Work out the finished part from the listing and answer in its coordinate system (mm). Face numbers are marked on the shaded views. Coordinates: 2 decimals unless noted, no trailing zeros. Write each loop counter-clockwise with the first axis right and the second up, starting at its lowest first coordinate (ties: lowest second). Pieces come first, ordered by that corner, then holes. Notation, with made-up numbers: (46, -24) - (66, -24) arc R21 ccw to (66, 12) - close; hole circle Ø6 at (0, 39). An arc over 180 degrees is marked (long way). One line per item, written item: value.
```python
from build123d import *

# Parameters (mm, degrees)
ESQUISSE1_W             = 92.6
ESQUISSE1_H             = 142.6
BASE_EXTRUSION_DEPTH    = 7
ESQUISSE4_R             = 1.6
ENL_V_MAT_EXTRU_2_DEPTH = 108.918117107
ESQUISSE2_W             = 79.5
ESQUISSE2_H             = 104
ENL_V_MAT_EXTRU_3_DEPTH = 4
ESQUISSE6_W             = 86.3
ESQUISSE6_H             = 9.5
ENL_V_MAT_EXTRU_4_DEPTH = 4
ESQUISSE7_W             = 120
ESQUISSE7_H             = 17.9
ENL_V_MAT_EXTRU_6_DEPTH = 4
ESQUISSE8_W             = 13.8
ESQUISSE8_H             = 8.9
ESQUISSE8_W_2           = 65.8
ENL_V_MAT_EXTRU_7_DEPTH = 15


with BuildPart() as part:
    # Esquisse1 → Base-Extrusion (new body)
    with BuildSketch(Plane.XY):
        with Locations((1.3, -25.3)):
            Rectangle(ESQUISSE1_W, ESQUISSE1_H)
    extrude(amount=BASE_EXTRUSION_DEPTH)

    # Esquisse4 → Enlèv. mat.-Extru.2 (cut, through all)
    with BuildSketch(Plane.XY.offset(7)):
        with Locations((-30.2, 44)):
            Circle(ESQUISSE4_R)
        with Locations((43.6, 44)):
            Circle(ESQUISSE4_R)
        with Locations((-30.2, -94.6)):
            Circle(ESQUISSE4_R)
        with Locations((43.6, -94.6)):
            Circle(ESQUISSE4_R)
    extrude(amount=-ENL_V_MAT_EXTRU_2_DEPTH, mode=Mode.SUBTRACT)

    # Esquisse2 → Enlèv. mat.-Extru.3 (cut)
    with BuildSketch(Plane.XY.offset(7)):
        with Locations((5.05, -15.3)):
            Rectangle(ESQUISSE2_W, ESQUISSE2_H)
    extrude(amount=-ENL_V_MAT_EXTRU_3_DEPTH, mode=Mode.SUBTRACT)

    # Esquisse6 → Enlèv. mat.-Extru.4 (cut)
    with BuildSketch(Plane.XY.offset(7)):
        with Locations((7.85, 44.25)):
            Rectangle(ESQUISSE6_W, ESQUISSE6_H)
    extrude(amount=-ENL_V_MAT_EXTRU_4_DEPTH, mode=Mode.SUBTRACT)

    # Esquisse7 → Enlèv. mat.-Extru.6 (cut)
    with BuildSketch(Plane.XY.offset(7)):
        with Locations((0, -99.05)):
            Rectangle(ESQUISSE7_W, ESQUISSE7_H)
    extrude(amount=-ENL_V_MAT_EXTRU_6_DEPTH, mode=Mode.SUBTRACT)

    # Esquisse8 → Enlèv. mat.-Extru.7 (cut)
    with BuildSketch(Plane(origin=(0, 0, 0), x_dir=(-1, 0, 0), z_dir=(0, 0, -1))):
        with Locations((41.1, -94.55)):
            Rectangle(ESQUISSE8_W, ESQUISSE8_H)
        with Locations((-6.7, -94.55)):
            Rectangle(ESQUISSE8_W_2, ESQUISSE8_H)
    extrude(amount=-ENL_V_MAT_EXTRU_7_DEPTH, mode=Mode.SUBTRACT)


solid = part.part
```
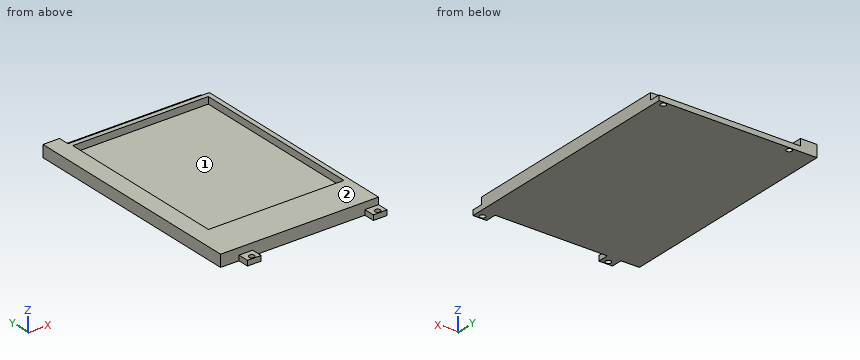
Item 1: Section D-D, the plane z = 1.75 is taken. Determine the outline of the cut face in (x, y), then the cut area to 3 significant figures.
Evaluation:
outline: (-45, -90.1) - (-34.2, -90.1) - (-34.2, -96.6) - (-26.2, -96.6) - (-26.2, -90.1) - (39.6, -90.1) - (39.6, -96.6) - (47.6, -96.6) - (47.6, 46) - (-45, 46) - close; hole circle Ø3.2 at (-30.2, -94.6); hole circle Ø3.2 at (-30.2, 44); hole circle Ø3.2 at (43.6, -94.6); hole circle Ø3.2 at (43.6, 44)
area: 12,700 mm2
Item 2: Section A-A, the plane y = -94.6 is taken. Determine the outline of the cut face in (x, z), then the cut area to 3 significant figures.
Evaluation:
outline: (-34.2, 0) - (-31.8, 0) - (-31.8, 3) - (-34.2, 3) - close; (-28.6, 0) - (-26.2, 0) - (-26.2, 3) - (-28.6, 3) - close; (39.6, 0) - (42, 0) - (42, 3) - (39.6, 3) - close; (45.2, 0) - (47.6, 0) - (47.6, 3) - (45.2, 3) - close
area: 28.8 mm2
Item 3: Given pin 1 (6 mm diameter, centred on x = -31, y = -44.5, fed in from +Z); pin 2 (1.2 mm diameter, centred on x = -6.5, z = 4.5, fed in from +Y); pin 3 (1.5 mm diameter, centred on y = -93, z = 1, fed in from -X), each flat-ended and moving along its own axis, determine where each tip first touches the part or whether it passes through.
Evaluation:
pin 1: stops at z = 3
pin 2: stops at y = 39.5
pin 3: stops at x = -34.2
Item 4: Section B-B, the plane y = 44 is taken. Determine the outline of the cut face in (x, z).
Evaluation:
outline: (-45, 0) - (-31.8, 0) - (-31.8, 3) - (-35.3, 3) - (-35.3, 7) - (-45, 7) - close; (-28.6, 0) - (42, 0) - (42, 3) - (-28.6, 3) - close; (45.2, 0) - (47.6, 0) - (47.6, 3) - (45.2, 3) - close
Item 5: Consider probe 1 along Y at (x, z) = (-30.2, 2.1); probe 2 along X at (y, z) = (-94.6, 0.7); probe 3 along X at (y, z) = (28, 6.5). Determine where each line is inside the solid, lowest interval first.
Evaluation:
probe 1: y = -96.6 to -96.2, -93 to 42.4, 45.6 to 46
probe 2: x = -34.2 to -31.8, -28.6 to -26.2, 39.6 to 42, 45.2 to 47.6
probe 3: x = -45 to -34.7, 44.8 to 47.6
Item 6: Determine the mould class of the marked faces 1 and 2 for opening direction X: +X half, -X half, draft (parallel to the pull), parting line (faces both ways), or undercut.
Evaluation:
face 1: undercut
face 2: draft
Item 7: Section C-C, the plane x = 22 is taken. Determine the outline of the cut face in (y, z), then the cut area to 3 significant figures.
Evaluation:
outline: (-90.1, 0) - (46, 0) - (46, 3) - (39.5, 3) - (39.5, 7) - (36.7, 7) - (36.7, 3) - (-67.3, 3) - (-67.3, 7) - (-90.1, 7) - close
area: 511 mm2
